Here's how the part is built. I have some questions about the finished solid (model axes, mm). Coordinates: 2 decimals unless noted, no trailing zeros. Write each loop counter-clockwise with the first axis right and the second up, starting at its lowest first coordinate (ties: lowest second). Pieces come first, ordered by that corner, then holes. Notation, with made-up numbers: (80, 77) - (111, 77) arc R37 ccw to (111, 113) - close; hole circle Ø11 at (60.25, -32.75). An arc over 180 degrees is marked (long way). Answer in a Markdown table with one row per item. Add a question column.
Item 1: Imagine slicing it at B-B (y = -24). Please give me the cut outline in (x, z).
Item 2: Imagine slicing it at A-A (x = 2). Please give me the cut outline in (y, z).
Item 3: Imagine slicing it at C-C (x = 33.5). Please give me the cut outline in (y, z), plus the area to 4 significant figures.
Item 4: Imagine slicing it at D-D (y = -18). Please give me the cut outline in (x, z).
Item 5: I'm going to push flat-ended pins straight in: pin 1 (1.5 mm diameter, centred on y = 26, z = 3, fed in from +X); pin 2 (1.5 mm diameter, centred on x = 0, z = 2, fed in from -Y); pin 3 (1 mm diameter, centred on x = -26, z = 3.5, fed in from +Y). Where does each tip first touch, or does it pass through?
Item 6: If I drill on probe 1 along Y at (x, z) = (2.5, 2.2); probe 2 along Y at (x, z) = (17.5, 4.45); probe 3 along X at (y, z) = (25, 4.6), over which ranges is the centre line in solid material (lowest first)? Write a range as from..to.
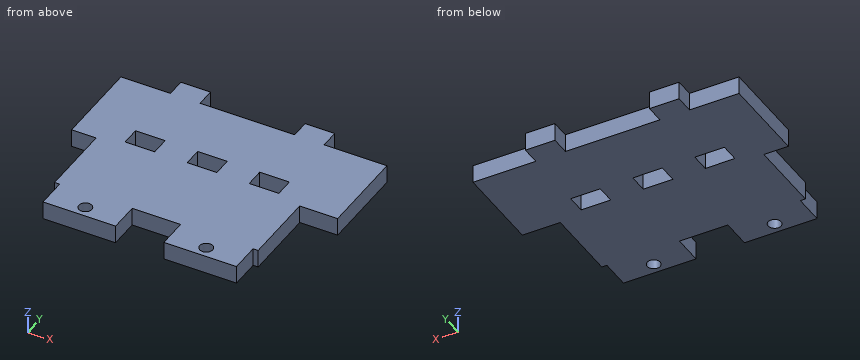
from build123d import *

# Parameters (mm, degrees)
BOSS_EXTRUDE1_DEPTH = 5
CUT_EXTRUDE1_REACH  = 7
SKETCH2_R           = 1.8
SKETCH2_W           = 8.2
SKETCH2_H           = 5.2
SKETCH3_W           = 3.7
SKETCH3_H           = 24.5
BOSS_EXTRUDE4_DEPTH = 5
SKETCH4_W           = 8.2
SKETCH4_H           = 5.2
BOSS_EXTRUDE7_DEPTH = 5


with BuildPart() as part:
    # Sketch1 → Boss-Extrude1 (new body)
    with BuildSketch(Plane.XY):
        Polygon((26.917617282, -2.091463415), (33.717617282, -2.091463415), (33.717617282, 22.408536585), (-36.282382718, 22.408536585), (-36.282382718, -2.091463415), (-29.482382718, -2.091463415), (-29.482382718, -22.691463415), (-28.082382718, -22.691463415), (-28.082382718, -30.955691057), (-7.982382718, -30.955691057), (-7.982382718, -22.691463415), (5.417617282, -22.691463415), (5.417617282, -30.955691057), (25.517617282, -30.955691057), (25.517617282, -22.691463415), (26.917617282, -22.691463415), align=None)
    extrude(amount=BOSS_EXTRUDE1_DEPTH)

    # Sketch2 → Cut-Extrude1 (cut, up to next)
    with BuildSketch(Plane.XY.offset(5), mode=Mode.PRIVATE) as cut_extrude1_sk1:
        with Locations((15.417617282, -27.855691057)):
            Circle(SKETCH2_R)
    cut_extrude1_tool1 = extrude(cut_extrude1_sk1.sketch, amount=-CUT_EXTRUDE1_REACH, mode=Mode.PRIVATE) & part.part
    add(cut_extrude1_tool1.solids().sort_by_distance((15.417617, -27.855691, 5))[0], mode=Mode.SUBTRACT)
    # Sketch2 → Cut-Extrude1 (cut, up to next)
    with BuildSketch(Plane.XY.offset(5), mode=Mode.PRIVATE) as cut_extrude1_sk2:
        with Locations((-18.082382718, -27.855691057)):
            Circle(SKETCH2_R)
    cut_extrude1_tool2 = extrude(cut_extrude1_sk2.sketch, amount=-CUT_EXTRUDE1_REACH, mode=Mode.PRIVATE) & part.part
    add(cut_extrude1_tool2.solids().sort_by_distance((-18.082383, -27.855691, 5))[0], mode=Mode.SUBTRACT)
    # Sketch2 → Cut-Extrude1 (cut, up to next)
    with BuildSketch(Plane.XY.offset(5), mode=Mode.PRIVATE) as cut_extrude1_sk3:
        with Locations((-18.482382718, 2.508536585)):
            Rectangle(SKETCH2_W, SKETCH2_H)
    cut_extrude1_tool3 = extrude(cut_extrude1_sk3.sketch, amount=-CUT_EXTRUDE1_REACH, mode=Mode.PRIVATE) & part.part
    add(cut_extrude1_tool3.solids().sort_by_distance((-18.482383, 2.508537, 5))[0], mode=Mode.SUBTRACT)
    # Sketch2 → Cut-Extrude1 (cut, up to next)
    with BuildSketch(Plane.XY.offset(5), mode=Mode.PRIVATE) as cut_extrude1_sk4:
        with Locations((-1.282382718, 2.508536585)):
            Rectangle(SKETCH2_W, SKETCH2_H)
    cut_extrude1_tool4 = extrude(cut_extrude1_sk4.sketch, amount=-CUT_EXTRUDE1_REACH, mode=Mode.PRIVATE) & part.part
    add(cut_extrude1_tool4.solids().sort_by_distance((-1.282383, 2.508537, 5))[0], mode=Mode.SUBTRACT)
    # Sketch2 → Cut-Extrude1 (cut, up to next)
    with BuildSketch(Plane.XY.offset(5), mode=Mode.PRIVATE) as cut_extrude1_sk5:
        with Locations((15.917617282, 2.508536585)):
            Rectangle(SKETCH2_W, SKETCH2_H)
    cut_extrude1_tool5 = extrude(cut_extrude1_sk5.sketch, amount=-CUT_EXTRUDE1_REACH, mode=Mode.PRIVATE) & part.part
    add(cut_extrude1_tool5.solids().sort_by_distance((15.917617, 2.508537, 5))[0], mode=Mode.SUBTRACT)

    # Sketch3 → Boss-Extrude4 (add)
    with BuildSketch(Plane.XY.offset(5)):
        with Locations((35.567617282, 10.158536585)):
            Rectangle(SKETCH3_W, SKETCH3_H)
    extrude(amount=-BOSS_EXTRUDE4_DEPTH)

    # Sketch4 → Boss-Extrude7 (add)
    with BuildSketch(Plane.XY.offset(5)):
        with Locations((-18.482382718, 25.008536585)):
            Rectangle(SKETCH4_W, SKETCH4_H)
        with Locations((15.917617282, 25.008536585)):
            Rectangle(SKETCH4_W, SKETCH4_H)
    extrude(amount=-BOSS_EXTRUDE7_DEPTH)


solid = part.part
Here are the results:
| question | item | result |
|---|---|---|
| 1 | outline | (-28.08, 0) - (-7.98, 0) - (-7.98, 5) - (-28.08, 5) - close; (5.42, 0) - (25.52, 0) - (25.52, 5) - (5.42, 5) - close |
| 2 | outline | (-22.69, 0) - (-0.09, 0) - (-0.09, 5) - (-22.69, 5) - close; (5.11, 0) - (22.41, 0) - (22.41, 5) - (5.11, 5) - close |
| 3 | outline | (-2.09, 0) - (22.41, 0) - (22.41, 5) - (-2.09, 5) - close |
| 3 | area | 122.5 mm2 |
| 4 | outline | (-29.48, 0) - (26.92, 0) - (26.92, 5) - (-29.48, 5) - close |
| 5 | pin 1 | stops at x = 20.02 |
| 5 | pin 2 | stops at y = -22.69 |
| 5 | pin 3 | stops at y = 22.41 |
| 6 | probe 1 | y = -22.69..-0.09, 5.11..22.41 |
| 6 | probe 2 | y = -30.96..-0.09, 5.11..27.61 |
| 6 | probe 3 | x = -22.58..-14.38, 11.82..20.02 |
